The listing builds one solid part. Answer for the finished solid, in the listing's coordinates (mm). Face numbers are marked on the shaded views. A direction names the side the tool comes from. Round coordinates to 2 decimals unless told otherwise and drop trailing zeros. Order: outer loops, then holes, each group sorted by start corner. A loop starts at its lowest first (then second) coordinate and runs counter-clockwise, first axis right, second up. Notation, with made-up numbers: (80, -21) - (86, -21) arc R34 cw to (86, 14) - close; hole circle Ø7 at (29, -21.5). An arc over 180 degrees is marked (long way). One line per item, written item: value. Start each with the question number.
1. Section D-D, the plane x = 13 is taken. Give the vertices of the cut face in (y, z), then the cut area to 3 significant figures.
2. Section A-A, the plane y = -6.5 is taken. Give the vertices of the cut face in (x, z), then the cut area to 3 significant figures.
3. Section B-B, the plane z = 25.5 is taken. Give the vertices of the cut face in (x, y).
4. Section C-C, the plane x = -10.5 is taken. Count the separate pieces of the cut face and the enclosed holes in it, then the cut area to 3 significant figures.
5. Flat-ended cylindrical pins translate along their axes: P1, Ø4, axis at x = 10.5, y = -6.5, coming from the +Z side; P2, Ø5.5, axis at x = -10.5, y = 8.5, coming from the -Z side. Find the tip coordinate at first contact, or state that the pin passes through.
6. A tool of negligible diameter and unlimited length cuts with its end or side. For the marked faces 4, 5 and 6, from which of +Z, -Z, +X, -X, +Y, -Y can it reach the whole face along a straight path? Write none if from no direction.
7. For a pull along Y with two mould halves and no side action, classify the marked faces 1, 2 and 3 as released by +Y, released by -Y, zero draft, split by the parting line, or undercut.
8. Straight lines are drawn through the part: line 1 (Y direction, x = -10.5, z = 0.75); line 2 (Y direction, x = -20, z = 69.5); line 3 (Z direction, x = -7, y = -6.5). For each, find the intervals that lie inside material, in ascending order.
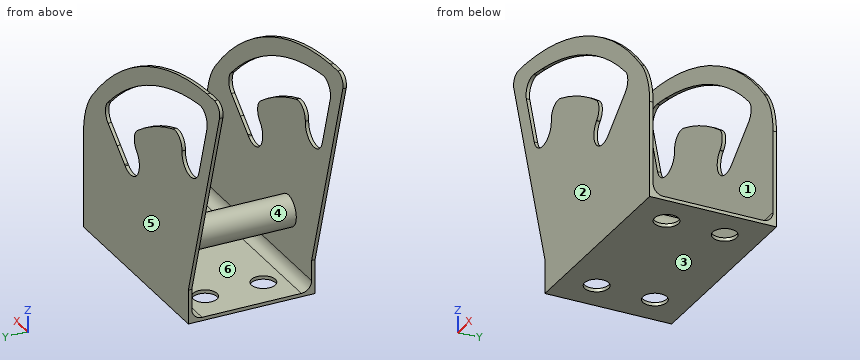
from build123d import *

# Parameters (mm, degrees)
CROQUIS1_W                   = 79
CROQUIS1_H                   = 35
SALIENTE_EXTRUIR1_DEPTH      = 1
SALIENTE_EXTRUIR3_DEPTH      = 72
SALIENTE_EXTRUIR3_DEPTH_BACK = 1
CROQUIS2_W                   = 79
CROQUIS2_H                   = 1
CORTAR_EXTRUIR1_DEPTH        = 72
CORTAR_EXTRUIR2_DEPTH        = 72
CORTAR_EXTRUIR3_DEPTH        = 72
REDONDEO4_R                  = 3
REDONDEO5_R                  = 20
REDONDEO6_R                  = 3
CORTAR_EXTRUIR4_DEPTH        = 72
REDONDEO7_START              = -18.5
REDONDEO7_DEPTH              = 1
REDONDEO7_2_DEPTH            = 1
REDONDEO8_R                  = 4
REDONDEO9_R                  = 3
CROQUIS8_R                   = 3.5
CORTAR_EXTRUIR5_DEPTH        = 72
CROQUIS13_R                  = 4.5
SALIENTE_EXTRUIR7_DEPTH      = 37


with BuildPart() as part:
    # Croquis1 → Saliente-Extruir1 (new body)
    with BuildSketch(Plane.XY):
        Rectangle(CROQUIS1_W, CROQUIS1_H)
    extrude(amount=SALIENTE_EXTRUIR1_DEPTH)

    # Croquis2 → Saliente-Extruir3 (add, two sides: drawn at the far end of the back side and taken through both)
    with BuildSketch(Plane.XY.offset(1).offset(-SALIENTE_EXTRUIR3_DEPTH_BACK)):
        with Locations((0, -18)):
            Rectangle(CROQUIS2_W, CROQUIS2_H)
        with Locations((0, 18)):
            Rectangle(CROQUIS2_W, CROQUIS2_H)
    extrude(amount=SALIENTE_EXTRUIR3_DEPTH + SALIENTE_EXTRUIR3_DEPTH_BACK)

    # Croquis3 → Cortar-Extruir1 (cut)
    with BuildSketch(Plane.XZ.offset(18.5)):
        Polygon((-39.5, 1), (-20.5, 1), (-20.5, 10), (-39.5, 73), align=None)
    extrude(amount=-CORTAR_EXTRUIR1_DEPTH, mode=Mode.SUBTRACT)

    # Croquis4 → Cortar-Extruir2 (cut)
    with BuildSketch(Plane.XY.offset(1)):
        Polygon((-20.5, 17.5), (-20.5, 18.5), (-39.5, 18.5), (-39.5, -18.5), (-20.5, -18.5), (-20.5, -17.5), align=None)
    extrude(amount=-CORTAR_EXTRUIR2_DEPTH, mode=Mode.SUBTRACT)

    # Croquis5 → Cortar-Extruir3 (cut)
    with BuildSketch(Plane.XZ.offset(18.5)):
        with BuildLine():
            ThreePointArc((-31.235435529, 73), (8.464348123, 62.063962298), (39.5, 35))
            Line((39.5, 35), (39.5, 73))
            Line((39.5, 73), (-31.235435529, 73))
        make_face()
    extrude(amount=-CORTAR_EXTRUIR3_DEPTH, mode=Mode.SUBTRACT)

    # Redondeo4
    redondeo4_edges = [part.edges().sort_by_distance(p)[0] for p in [
        (-39.5, -18, 73),
    ]]
    fillet(redondeo4_edges, radius=REDONDEO4_R)

    # Redondeo5
    redondeo5_edges = [part.edges().sort_by_distance(p)[0] for p in [
        (39.5, 18, 35),
        (39.5, -18, 35),
    ]]
    fillet(redondeo5_edges, radius=REDONDEO5_R)

    # Redondeo6
    redondeo6_edges = [part.edges().sort_by_distance(p)[0] for p in [
        (-39.5, 18, 73),
    ]]
    fillet(redondeo6_edges, radius=REDONDEO6_R)

    # Croquis6 → Cortar-Extruir4 (cut)
    with BuildSketch(Plane.XZ.offset(18.5)):
        with BuildLine():
            Line((16.016209597, 29.655049393), (16.02986755, 29.640967118))
            Line((16.02986755, 29.640967118), (20.305135111, 33.109993252))
            Line((20.305135111, 33.109993252), (20.307251231, 33.111710308))
            Line((20.307251231, 33.111710308), (28.870480014, 40.060062433))
            ThreePointArc((28.870480014, 40.060062433), (5.697385816, 57.873252637), (-22.045320516, 67.073485531))
            ThreePointArc((-22.045320516, 67.073485531), (-26.684583157, 67.660916613), (-31.348578825, 68))
            Line((-31.348578825, 68), (-32.769624166, 68))
            Line((-32.769624166, 68), (-26.623611491, 47.621115867))
            ThreePointArc((-26.623611491, 47.621115867), (-20.392867483, 44.277789814), (-17.049541429, 50.508533823))
            Line((-17.049541429, 50.508533823), (-18.465863192, 55.204758613))
            ThreePointArc((-18.465863192, 55.204758613), (-1.905942772, 49.399230787), (12.898781807, 39.978230428))
            ThreePointArc((12.898781807, 39.978230428), (12.954271862, 39.933178304), (13.009719865, 39.888074435))
            Line((13.009719865, 39.888074435), (9.803992697, 37.43240656))
            Line((9.803992697, 37.43240656), (9.202695315, 36.971797598))
            ThreePointArc((9.202695315, 36.971797598), (9.127703809, 36.903372112), (9.054116963, 36.833438221))
            ThreePointArc((9.054116963, 36.833438221), (8.795597311, 29.925261077), (15.685593651, 29.361617315))
            ThreePointArc((15.685593651, 29.361617315), (15.85414601, 29.504677838), (16.016209597, 29.655049393))
        make_face()
    extrude(amount=-CORTAR_EXTRUIR4_DEPTH, mode=Mode.SUBTRACT)

    # Redondeo7: read off the stored shape, not the designer's step
    # Redondeo7 outline → Redondeo7 (cut)
    with BuildSketch(Plane(origin=(0, 0, 0), x_dir=(1, 0, 0), z_dir=(0, 1, 0)).offset(REDONDEO7_START)):
        with BuildLine():
            ThreePointArc((9.143619043, -36.918128357), (10.421654669, -40.121349), (8.732679814, -43.12823468))
            ThreePointArc((8.732679814, -43.12823468), (10.899572634, -41.545606896), (13.009719865, -39.888074435))
            Line((13.009719865, -39.888074435), (9.202695315, -36.971797598))
            ThreePointArc((9.202695315, -36.971797598), (9.173050087, -36.945080858), (9.143619043, -36.918128357))
        make_face()
        with BuildLine():
            ThreePointArc((-18.465863192, -55.204758613), (-15.014619907, -54.339507434), (-11.607267341, -53.314964462))
            ThreePointArc((-11.607267341, -53.314964462), (-15.276738996, -52.690173302), (-16.842756461, -49.313344091))
            ThreePointArc((-16.842756461, -49.313344091), (-16.90977213, -49.917232668), (-17.049541429, -50.508533823))
            Line((-17.049541429, -50.508533823), (-18.465863192, -55.204758613))
        make_face()
    extrude(amount=REDONDEO7_DEPTH, mode=Mode.SUBTRACT)

    # Redondeo7 2 outline → Redondeo7 2 (add)
    with BuildSketch(Plane(origin=(0, 0, 0), x_dir=(1, 0, 0), z_dir=(0, 1, 0)).offset(REDONDEO7_START)):
        with BuildLine():
            ThreePointArc((25.466305511, -37.297856291), (26.941907185, -40.223913599), (25.735427009, -43.270816494))
            ThreePointArc((25.735427009, -43.270816494), (27.323511874, -41.685513114), (28.870480014, -40.060062433))
            Line((28.870480014, -40.060062433), (25.466305511, -37.297856291))
        make_face()
        with BuildLine():
            ThreePointArc((-26.909207237, -67.682994851), (-30.387237337, -66.239442173), (-31.124981113, -62.546709875))
            Line((-31.124981113, -62.546709875), (-32.769624166, -68))
            Line((-32.769624166, -68), (-31.348578825, -68))
            ThreePointArc((-31.348578825, -68), (-29.12687991, -67.869689367), (-26.909207237, -67.682994851))
        make_face()
    extrude(amount=REDONDEO7_2_DEPTH)

    # Redondeo8
    redondeo8_edges = [part.edges().sort_by_distance(p)[0] for p in [
        (-18.465863192, 18, 55.204758613),
        (28.870480014, 18, 40.060062433),
        (-32.769624166, 18, 68),
        (13.009719865, 18, 39.888074435),
    ]]
    fillet(redondeo8_edges, radius=REDONDEO8_R)

    # Redondeo9
    redondeo9_edges = [part.edges().sort_by_distance(p)[0] for p in [
        (9.5, -17.5, 1),
        (9.5, 17.5, 1),
    ]]
    fillet(redondeo9_edges, radius=REDONDEO9_R)

    # Croquis8 → Cortar-Extruir5 (cut)
    with BuildSketch(Plane(origin=(0, 0, 0), x_dir=(-1, 0, 0), z_dir=(0, 0, -1))):
        with Locations((10.5, 8.5)):
            Circle(CROQUIS8_R)
        with Locations((-29.5, 8.5)):
            Circle(CROQUIS8_R)
        with Locations((-29.5, -8.5)):
            Circle(CROQUIS8_R)
        with Locations((10.5, -8.5)):
            Circle(CROQUIS8_R)
    extrude(amount=-CORTAR_EXTRUIR5_DEPTH, mode=Mode.SUBTRACT)

    # Croquis13 → Saliente-Extruir7 (add)
    with BuildSketch(Plane(origin=(0, 18.5, 0), x_dir=(1, 0, 0), z_dir=(0, 1, 0))):
        with Locations(Location((-7.199736414, -18.491822177, 0), (0, 0, 90))):
            Circle(CROQUIS13_R)
    extrude(amount=-SALIENTE_EXTRUIR7_DEPTH)


solid = part.part
Answer list:
1. outline: (-18.5, 0) - (18.5, 0) - (18.5, 28.27) - (17.5, 28.27) - (17.5, 4) arc R3 cw to (14.5, 1) - (-14.5, 1) arc R3 cw to (-17.5, 4) - (-17.5, 28.27) - (-18.5, 28.27) - close; (-18.5, 53.53) - (-17.5, 53.53) - (-17.5, 59.46) - (-18.5, 59.46) - close; (17.5, 53.53) - (18.5, 53.53) - (18.5, 59.46) - (17.5, 59.46) - close
1. area: 107 mm²
2. outline: (-20.5, 0) - (-13.37, 0) - (-13.37, 1) - (-20.5, 1) - close; circle Ø9 at (-7.2, 18.49); (-7.63, 0) - (26.63, 0) - (26.63, 1) - (-7.63, 1) - close; (32.37, 0) - (39.5, 0) - (39.5, 1) - (32.37, 1) - close
2. area: 112 mm²
3. outline: (-25.17, -18.5) - (39.5, -18.5) - (39.5, -17.5) - (-25.17, -17.5) - close; (-25.17, 17.5) - (39.5, 17.5) - (39.5, 18.5) - (-25.17, 18.5) - close
4. separate pieces: 4
4. enclosed holes: 0
4. area: 355 mm²
5. P1: stops at z = 1
5. P2: stops at z = 14.03
6. face 4: none
6. face 5: +Z, -Z, +X, -X, +Y
6. face 6: +X, -X
7. face 1: undercut
7. face 2: released by -Y
7. face 3: zero draft
8. line 1: y = -18.5 to -12, -5 to 5, 12 to 18.5
8. line 2: y = -18.5 to -17.5, 17.5 to 18.5
8. line 3: z = 0 to 1, 14 to 22.99
